Can you work these out from the model? Positions are in its coordinate system, mm. Face numbers are marked on the shaded views. A direction names the side the tool comes from. Round coordinates to 2 decimals unless told otherwise and drop trailing zeros. Loops run counter-clockwise (first coordinate to the right, second up) from the corner with the lowest first, then second, coordinate; pieces in that order, holes last.
from build123d import *

# Parameters (mm, degrees)
SKETCH1_W           = 2.5
SKETCH1_H           = 9
SKETCH1_W_2         = 4.5
SKETCH1_H_2         = 15
BOSS_EXTRUDE1_DEPTH = 4.5
FILLET1_R           = 5


with BuildPart() as part:
    # Sketch1 → Boss-Extrude1 (new body)
    with BuildSketch(Plane.XY):
        Polygon((-2.25, -15), (-2.25, 0), (-2.25, 15), (-25, 15), (-25, -15), (-22.5, -15), align=None)
        Polygon((2.25, 15), (2.25, 0), (2.25, -15), (22.5, -15), (25, -15), (25, 15), align=None)
        with Locations((-23.75, -19.5)):
            Rectangle(SKETCH1_W, SKETCH1_H)
        with Locations((23.75, -19.5)):
            Rectangle(SKETCH1_W, SKETCH1_H)
        with Locations((0, 7.5)):
            Rectangle(SKETCH1_W_2, SKETCH1_H_2)
    extrude(amount=BOSS_EXTRUDE1_DEPTH)

    # Fillet1
    fillet1_edges = [part.edges().sort_by_distance(p)[0] for p in [
        (-25, 15, 2.25),
        (25, 15, 2.25),
    ]]
    fillet(fillet1_edges, radius=FILLET1_R)


solid = part.part
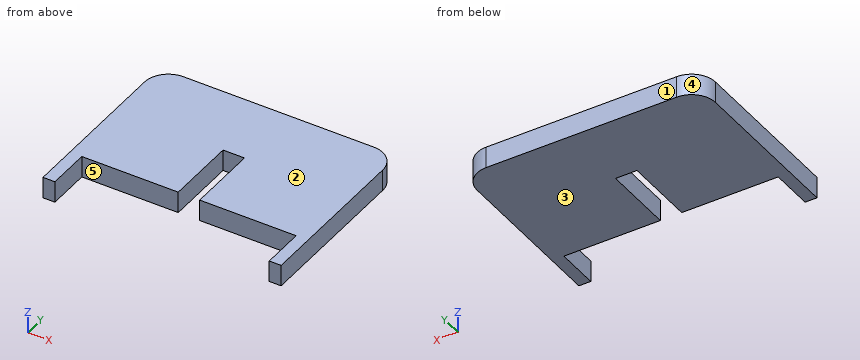
(1) If we mould it in two halves opening along Z, with no side actions, what happens to the marked faces 1, 2 and 3? For each: released by +Z, released by -Z, zero draft, split by the parting line, or undercut.
Worked answers:
face 1: zero draft
face 2: released by +Z
face 3: released by -Z
(2) If we section it at B-B, the plane z = 2.85: List the corners of the cut face in (x, y) for me.
Worked answers:
outline: (-25, -24) - (-22.5, -24) - (-22.5, -15) - (-2.25, -15) - (-2.25, 0) - (2.25, 0) - (2.25, -15) - (22.5, -15) - (22.5, -24) - (25, -24) - (25, 10) arc R5 ccw to (20, 15) - (-20, 15) arc R5 ccw to (-25, 10) - close
(3) For the marked faces 4 and 5, which set-ups out of +Z, -Z, +X, -X, +Y, -Y let a thin tool reach every point of the face, with its end or its side?
Worked answers:
face 4: +Z, -Z, -X, +Y
face 5: +Z, -Z, -Y
(4) If we section it at A-A, the plane y = -6.5: List the corners of the cut face in (x, z) for me.
Worked answers:
outline: (-25, 0) - (-2.25, 0) - (-2.25, 4.5) - (-25, 4.5) - close; (2.25, 0) - (25, 0) - (25, 4.5) - (2.25, 4.5) - close
(5) If we section it at D-D, the plane x = 8: List the corners of the cut face in (y, z) for me, then the cut area to 3 significant figures.
Worked answers:
outline: (-15, 0) - (15, 0) - (15, 4.5) - (-15, 4.5) - close
area: 135 mm2
(6) If I drill on line 1 (X direction, y = -13.5, z = 2); line 2 (X direction, y = -21.5, z = 3.55); line 3 (Y direction, x = 0, z = 3.9), over which ranges is the centre line in solid material (lowest first)?
Worked answers:
line 1: x = -25 to -2.25, 2.25 to 25
line 2: x = -25 to -22.5, 22.5 to 25
line 3: y = 0 to 15
(7) Will these pins go through, and if not, where does the flat tip stop? P1, Ø2, axis at x = -1, y = -2.5, coming from the -Z side; P2, Ø1.3, axis at x = 1, z = 1, coming from the -Y side.
Worked answers:
P1: passes through
P2: stops at y = 0
(8) If we section it at C-C, the plane x = -1: List the corners of the cut face in (y, z) for me.
Worked answers:
outline: (0, 0) - (15, 0) - (15, 4.5) - (0, 4.5) - close
